from build123d import *

# Parameters (mm, degrees)
SKETCH2_W         = 6
SKETCH2_H         = 6.1
COG_DEPTH         = 11.50809212
PATTERN_COG_COUNT = 16
SKETCH8_W         = 17.303989153
SKETCH8_H         = 4


with BuildPart() as part:
    # Sketch2 → Body (revolve)
    with BuildSketch(Plane.XY, mode=Mode.PRIVATE) as body_sk:
        with Locations((3, 3.05)):
            Rectangle(SKETCH2_W, SKETCH2_H)
    revolve(body_sk.sketch.rotate(Axis((0, 0, 0), (1, 0, 0)), 90), axis=Axis((0, 0, 0), (1, 0, 0)))

    # Sketch6 → Cog (cut, through all)
    with BuildSketch(Plane(origin=(0, 0, 0), x_dir=(0, 0, -1), z_dir=(1, 0, 0))):
        with BuildLine():
            Line((0.789835397, 5.82877936), (0.508392514, 5.225223151))
            ThreePointArc((0.508392514, 5.225223151), (0.429351309, 5.137842761), (0.314832372, 5.1101253))
            ThreePointArc((0.314832372, 5.1101253), (0, 5.11981445), (-0.314832372, 5.1101253))
            ThreePointArc((-0.314832372, 5.1101253), (-0.429351309, 5.137842761), (-0.508392514, 5.225223151))
            Line((-0.508392514, 5.225223151), (-0.789835397, 5.82877936))
            ThreePointArc((-0.789835397, 5.82877936), (-0.924476923, 5.968756351), (-1.116644684, 5.996924599))
            ThreePointArc((-1.116644684, 5.996924599), (0, 6.1), (1.116644684, 5.996924599))
            ThreePointArc((1.116644684, 5.996924599), (0.924476923, 5.968756351), (0.789835397, 5.82877936))
        make_face()
    cog = extrude(amount=COG_DEPTH, mode=Mode.SUBTRACT)

    # Pattern-Cog: Cog ×16 about axis
    pattern_cog_axis = Axis((0, 0, 0), (1, 0, 0))
    for i in range(1, PATTERN_COG_COUNT):
        add(cog.rotate(pattern_cog_axis, i * 360 / PATTERN_COG_COUNT), mode=Mode.SUBTRACT)

    # Sketch8 → Hole-Shaft (revolve, cut)
    with BuildSketch(Plane.XY, mode=Mode.PRIVATE) as hole_shaft_sk:
        with Locations((7.348005424, -2)):
            Rectangle(SKETCH8_W, SKETCH8_H)
    revolve(hole_shaft_sk.sketch.rotate(Axis((-1.303989153, 0, 0), (1, 0, 0)), 270), axis=Axis((-1.303989153, 0, 0), (1, 0, 0)), mode=Mode.SUBTRACT)


solid = part.part
Here's how the part is built. I have some questions about the finished solid (model axes, mm). Round coordinates to 2 decimals unless told otherwise and drop trailing zeros. Loops run counter-clockwise (first coordinate to the right, second up) from the corner with the lowest first, then second, coordinate; pieces in that order, holes last. Notation, with made-up numbers: (-21.75, 85.5) -> (7.25, 85.5) arc R27 cw to (7.25, 115.5) -> close; hole circle Ø1 at (22, 65). An arc over 180 degrees is marked (long way). Write each question's results on one line, items separated by ' | '.
(1) If we section it at A-A, the plane z = 0: List the corners of the cut face in (x, y) for me.
Worked answers:
outline: (0, -5.12) -> (6, -5.12) -> (6, -4) -> (0, -4) -> close; (0, 4) -> (6, 4) -> (6, 5.12) -> (0, 5.12) -> close
(2) If I drill on L1, parallel to Y at x = 1.75, z = 0; L2, parallel to Z at x = 3.5, y = -2.5; L3, parallel to Y at x = 2, z = -2.25, over which ranges is the centre line in solid material (lowest first)?
Worked answers:
L1: -5.12 to -4, 4 to 5.12 | L2: -4.66 to -3.12, 3.12 to 4.66 | L3: -4.6 to -3.31, 3.31 to 4.6
(3) For P1, Ø1, axis at x = 2.5, z = -4.5, coming from the +Y side, with a flat end and sliding along its axis, tell me the tip position at first contact or that it passes through.
Worked answers:
P1: y = 3.58
